Work out the finished part from the listing and answer in its coordinate system (mm). A direction names the side the tool comes from. Coordinates: 2 decimals unless noted, no trailing zeros. Order: outer loops, then holes, each group sorted by start corner. A loop starts at its lowest first (then second) coordinate and runs counter-clockwise, first axis right, second up. Notation, with made-up numbers: M 40,37.5 L 50,37.5 A13 ccw 50,51.5 Z; hole C -12.5,85 d7. An arc over 180 degrees is marked long. Use a Markdown table: item, result.
from build123d import *

# Parameters (mm, degrees)
SKETCH1_R           = 52.5
SKETCH1_R_2         = 40.5
SKETCH1_R_3         = 23.665
SKETCH1_R_4         = 11.665
BOSS_EXTRUDE1_DEPTH = 12
SKETCH1_3_R         = 23.665
SKETCH1_3_R_2       = 11.665
SKETCH1_3_R_3       = 52.5
SKETCH1_3_R_4       = 40.5
BOSS_EXTRUDE2_DEPTH = 25
SKETCH1_4_R         = 52.5
SKETCH1_4_R_2       = 40.5
BOSS_EXTRUDE3_DEPTH = 63
CUT_EXTRUDE1_DEPTH  = 3
FILLET1_R           = 3
FILLET2_R           = 3


with BuildPart() as part:
    # Sketch1 → Boss-Extrude1 (new body)
    with BuildSketch(Plane(origin=(0, 0, 0), x_dir=(1, 0, 0), z_dir=(0, 1, 0))):
        with BuildLine():
            Line((-17.301, 49.56738241), (-95.298631714, 22.343087709))
            ThreePointArc((-95.298631714, 22.343087709), (-73.798218994, 19.29490664), (-63.835, 0))
            ThreePointArc((-63.835, 0), (-73.798218994, -19.29490664), (-95.298631714, -22.343087709))
            Line((-95.298631714, -22.343087709), (-17.301, -49.56738241))
            ThreePointArc((-17.301, -49.56738241), (-52.5, 0), (-17.301, 49.56738241))
        make_face()
        with BuildLine():
            Line((95.298631714, 22.343087709), (17.301, 49.56738241))
            ThreePointArc((17.301, 49.56738241), (42.805096075, 30.396936523), (52.5, 0))
            ThreePointArc((52.5, 0), (42.805096075, -30.396936523), (17.301, -49.56738241))
            Line((17.301, -49.56738241), (95.298631714, -22.343087709))
            ThreePointArc((95.298631714, -22.343087709), (63.835, 0), (95.298631714, 22.343087709))
        make_face()
        Circle(SKETCH1_R)
        Circle(SKETCH1_R_2, mode=Mode.SUBTRACT)
        with Locations((87.5, 0)):
            Circle(SKETCH1_R_3)
        with Locations((87.5, 0)):
            Circle(SKETCH1_R_4, mode=Mode.SUBTRACT)
        with Locations((-87.5, 0)):
            Circle(SKETCH1_R_3)
        with Locations((-87.5, 0)):
            Circle(SKETCH1_R_4, mode=Mode.SUBTRACT)
    extrude(amount=BOSS_EXTRUDE1_DEPTH)

    # Sketch1_3 → Boss-Extrude2 (add)
    with BuildSketch(Plane(origin=(0, 0, 0), x_dir=(1, 0, 0), z_dir=(0, 1, 0))):
        with Locations((-87.5, 0)):
            Circle(SKETCH1_3_R)
        with Locations((-87.5, 0)):
            Circle(SKETCH1_3_R_2, mode=Mode.SUBTRACT)
        with Locations((87.5, 0)):
            Circle(SKETCH1_3_R)
        with Locations((87.5, 0)):
            Circle(SKETCH1_3_R_2, mode=Mode.SUBTRACT)
        Circle(SKETCH1_3_R_3)
        Circle(SKETCH1_3_R_4, mode=Mode.SUBTRACT)
    extrude(amount=BOSS_EXTRUDE2_DEPTH)

    # Sketch1_4 → Boss-Extrude3 (add)
    with BuildSketch(Plane(origin=(0, 0, 0), x_dir=(1, 0, 0), z_dir=(0, 1, 0))):
        Circle(SKETCH1_4_R)
        Circle(SKETCH1_4_R_2, mode=Mode.SUBTRACT)
    extrude(amount=BOSS_EXTRUDE3_DEPTH)

    # Sketch2 → Cut-Extrude1 (cut)
    with BuildSketch(Plane(origin=(0, 12, 0), x_dir=(1, 0, 0), z_dir=(0, 1, 0))):
        with BuildLine():
            Line((-78.3996229, -25.064025248), (-40.010112847, -38.46350049))
            ThreePointArc((-40.010112847, -38.46350049), (-55.5, 0), (-40.010112847, 38.46350049))
            Line((-40.010112847, 38.46350049), (-78.3996229, 25.064025248))
            ThreePointArc((-78.3996229, 25.064025248), (-60.835, 0), (-78.3996229, -25.064025248))
        make_face()
        with BuildLine():
            Line((78.3996229, 25.064025248), (40.010112847, 38.46350049))
            ThreePointArc((40.010112847, 38.46350049), (55.5, 0), (40.010112847, -38.46350049))
            Line((40.010112847, -38.46350049), (78.3996229, -25.064025248))
            ThreePointArc((78.3996229, -25.064025248), (60.835, 0), (78.3996229, 25.064025248))
        make_face()
    extrude(amount=-CUT_EXTRUDE1_DEPTH, mode=Mode.SUBTRACT)

    # Fillet1
    fillet1_edges = [part.edges().sort_by_distance(p)[0] for p in [
        (-78.3996229, 10.5, 25.064025248),
        (-78.3996229, 10.5, -25.064025248),
        (-40.010112847, 10.5, -38.46350049),
        (-40.010112847, 10.5, 38.46350049),
    ]]
    fillet(fillet1_edges, radius=FILLET1_R)

    # Fillet2
    fillet2_edges = [part.edges().sort_by_distance(p)[0] for p in [
        (78.3996229, 10.5, -25.064025248),
        (78.3996229, 10.5, 25.064025248),
        (40.010112847, 10.5, 38.46350049),
        (40.010112847, 10.5, -38.46350049),
    ]]
    fillet(fillet2_edges, radius=FILLET2_R)


solid = part.part
(1) Given P1, Ø14, axis at x = 87.5, z = 0, coming from the -Y side; P2, Ø8.5, axis at x = -61, z = 17, coming from the +Y side; P3, Ø14, axis at x = -89, z = 11, coming from the +Y side; P4, Ø4, axis at y = 24, z = 36.5, coming from the -X side, each flat-ended and moving along its own axis, determine where each tip first touches the part or whether it passes through.
Conclusion:
| item | result |
|---|---|
| P1 | through |
| P2 | y = 9 |
| P3 | y = 25 |
| P4 | x = -39.57 |
(2) Straight lines are drawn through the part: L1, parallel to X at y = 24, z = 0 (3 decimals); L2, parallel to Z at x = 87, y = 13; L3, parallel to X at y = 33, z = 0. For each, find the intervals that lie inside material, in ascending order.
Conclusion:
| item | result |
|---|---|
| L1 | -111.165 to -99.165, -75.835 to -63.835, -52.5 to -40.5, 40.5 to 52.5, 63.835 to 75.835, 99.165 to 111.165 |
| L2 | -23.66 to -11.65, 11.65 to 23.66 |
| L3 | -52.5 to -40.5, 40.5 to 52.5 |
(3) A cutting plane is placed at B-B (z = 0). Give the number of separate pieces and of enclosed holes in the cut face, then the cut area to 3 significant figures.
Conclusion:
| item | result |
|---|---|
| separate pieces | 4 |
| enclosed holes | 0 |
| area | 2,950 mm2 |
(4) Which of the six approach directions +Z, -Z, +X, -X, +Y, -Y give full straight-line access (tool end or side, diameter ignored) to faces 1 (the flat face through (-98.3, 25, 4.9)), 2 (the cylindrical face through (-82.12, 12.32, 10.35)), 3 (the flat face through (60.664, 10.521, 31.255)), 4 (the flat face through (76.7, 25, 4.9))?
Conclusion:
| item | result |
|---|---|
| face 1 | +Z, -Z, -X, +Y |
| face 2 | +Y, -Y |
| face 3 | +Y |
| face 4 | +Z, -Z, +X, +Y |
(5) A cutting plane is placed at A-A (x = 0). Determine the outline of the cut face in (y, z).
Conclusion:
| item | result |
|---|---|
| outline | M 0,-52.5 L 63,-52.5 L 63,-40.5 L 0,-40.5 Z; M 0,40.5 L 63,40.5 L 63,52.5 L 0,52.5 Z |
(6) A cutting plane is placed at C-C (y = 46.5). Determine the outline of the cut face in (x, z), then the cut area to 3 significant figures.
Conclusion:
| item | result |
|---|---|
| outline | C 0,0 d105; hole C 0,0 d81 |
| area | 3,510 mm2 |
(7) A cutting plane is placed at D-D (x = -87.5). Determine the outline of the cut face in (y, z) (3 decimals).
Conclusion:
| item | result |
|---|---|
| outline | M 0,-25.065 L 12,-25.065 L 12,-23.665 L 25,-23.665 L 25,-11.665 L 0,-11.665 Z; M 0,11.665 L 25,11.665 L 25,23.665 L 12,23.665 L 12,25.065 L 0,25.065 Z |
